from build123d import *

# Parameters (mm, degrees)
SKETCH_W     = 37
SKETCH_H     = 12
SKETCH_R     = 0.9
PAD_DEPTH    = 7
SKETCH001_W  = 20.5
SKETCH001_H  = 12
POCKET_DEPTH = 3.5
FILLET_R     = 2


with BuildPart() as part:
    # Sketch → Pad (new body)
    with BuildSketch(Plane.XY):
        with Locations((8.5, 0)):
            Rectangle(SKETCH_W, SKETCH_H)
        with Locations((12, 0)):
            Circle(SKETCH_R, mode=Mode.SUBTRACT)
        with Locations((21, 0)):
            Circle(SKETCH_R, mode=Mode.SUBTRACT)
        with BuildLine():
            ThreePointArc((-3, 2.1), (-5.1, 0), (-3, -2.1))
            Line((-3, -2.1), (3, -2.1))
            ThreePointArc((3, -2.1), (5.1, 0), (3, 2.1))
            Line((-3, 2.1), (3, 2.1))
        make_face(mode=Mode.SUBTRACT)
    extrude(amount=PAD_DEPTH)

    # Sketch001 → Pocket (cut)
    with BuildSketch(Plane.XY):
        with Locations((16.75, 0)):
            Rectangle(SKETCH001_W, SKETCH001_H)
    extrude(amount=POCKET_DEPTH, mode=Mode.SUBTRACT)

    # Fillet
    fillet_edges = [part.edges().sort_by_distance(p)[0] for p in [
        (27, 6, 5.25),
        (27, -6, 5.25),
        (-10, -6, 3.5),
        (-10, 6, 3.5),
    ]]
    fillet(fillet_edges, radius=FILLET_R)


solid = part.part
Verification items for the finished model (mm, model axes). A direction names the side the tool comes from. Give positions to 0.01 mm unless a question says otherwise; leave off trailing zeros. Write each loop counter-clockwise with the first axis right and the second up, starting at its lowest first coordinate (ties: lowest second). Pieces come first, ordered by that corner, then holes. Notation, with made-up numbers: M 46,52.5 L 66,52.5 A37 ccw 66,88.5 Z; hole C -30,79.5 d10. An arc over 180 degrees is marked long. Put each result on its own line as item: value. Start each with the question number.
1. Section check B-B (z = 1). Record the cut outline in (x, y), and give its area (3 significant figures).
2. Section check A-A (x = 12). Record the cut outline in (y, z), and give its area (3 significant figures).
3. Set-up check for faces 4 (the face through (17, 0, 3.5)), 5 (the face through (5.1, 0, 3.5)), 6 (the face through (26.4, -5.43, 5.27)): record each of +Z, -Z, +X, -X, +Y, -Y from which the full face is reachable in a straight line by a thin tool's end or side.
4. Draft check along Y on faces 1 (the face through (-9.43, -5.4, 3.55)), 2 (the face through (-9.43, 5.4, 3.55)), 3 (the face through (-5.1, 0, 3.5)). Enter one of: +Y half, -Y half, draft (parallel to the pull), parting line (faces both ways), or undercut.
5. Scan lines: line 1 along X through (y, z) = (0, 5.45); line 2 along Y through (x, z) = (-3, 4); line 3 along Y through (x, z) = (12, 4.4). Record each from-to range of solid material in increasing order. Write a range as [from, to].
6. Go/stop test with flat-tipped pins: pin 1 Ø2 at (x, y) = (13, -3.5) entering from -Z; pin 2 Ø2 at (x, y) = (21, 0) entering from +Z; pin 3 Ø1 at (y, z) = (-0.5, 1.5) entering from +X. Record where each tip stops, or that it passes through.
7. Section check C-C (y = 0). Record the cut outline in (x, z).
8. Section check D-D (z = 5). Record the cut outline in (x, y), and give its area (3 significant figures).
Answer list:
1. outline: M -10,-4 A2 ccw -8,-6 L 6.5,-6 L 6.5,6 L -8,6 A2 ccw -10,4 Z; hole M -3,-2.1 L 3,-2.1 A2.1 ccw 3,2.1 L -3,2.1 A2.1 ccw Z
1. area: 157 mm2
2. outline: M -6,3.5 L -0.9,3.5 L -0.9,7 L -6,7 Z; M 0.9,3.5 L 6,3.5 L 6,7 L 0.9,7 Z
2. area: 35.7 mm2
3. face 4: -Z, +X, +Y, -Y
3. face 5: +Z, -Z
3. face 6: +Z, -Z, +X, -Y
4. face 1: -Y half
4. face 2: +Y half
4. face 3: undercut
5. line 1: [-10, -5.1], [5.1, 11.1], [12.9, 20.1], [21.9, 27]
5. line 2: [-6, -2.1], [2.1, 6]
5. line 3: [-6, -0.9], [0.9, 6]
6. pin 1: z = 3.5
6. pin 2: z = 7
6. pin 3: x = 6.5
7. outline: M -10,0 L -5.1,0 L -5.1,7 L -10,7 Z; M 5.1,0 L 6.5,0 L 6.5,3.5 L 11.1,3.5 L 11.1,7 L 5.1,7 Z; M 12.9,3.5 L 20.1,3.5 L 20.1,7 L 12.9,7 Z; M 21.9,3.5 L 27,3.5 L 27,7 L 21.9,7 Z
8. outline: M -10,-4 A2 ccw -8,-6 L 25,-6 A2 ccw 27,-4 L 27,4 A2 ccw 25,6 L -8,6 A2 ccw -10,4 Z; hole M -3,-2.1 L 3,-2.1 A2.1 ccw 3,2.1 L -3,2.1 A2.1 ccw Z; hole C 12,0 d1.8; hole C 21,0 d1.8
8. area: 396 mm2
